Input: part model. Units: mm. Frame: model coordinates. A direction names the side the tool comes from. Round coordinates to 2 decimals unless told otherwise and drop trailing zeros. Write each loop counter-clockwise with the first axis right and the second up, starting at its lowest first coordinate (ties: lowest second). Pieces come first, ordered by that corner, then holes. Notation, with made-up numbers: (85, 24.25) -> (99, 24.25) arc R24 cw to (99, 52.25) -> close; hole circle Ø7 at (10.5, 23.5). An arc over 180 degrees is marked (long way). Write item = value, one per line.
Solid Edge part; units mm, degrees
sketch "Sketch1" plane through (0, 0, 0) normal (1, 0, 0) x (0, 1, 0)
  circle A0 centre (0, 0) radius 2.5
extrude "Protrusion1" add sketch "Sketch1" along normal mid plane 40
sketch "Sketch2" plane through (0, 0, 0) normal (0, -1, 0) x (1, 0, 0)
  line L0 (30, 0) -> (30, 20)
  line L1 (30, -10) -> (30, 0)
  line L2 (20, -10) -> (30, -10)
  line L3 (20, 20) -> (20, -10)
  line L4 (20, 20) -> (-20, 20)
  line L5 (-20, -10) -> (-20, 20)
  line L6 (-30, -10) -> (-20, -10)
  line L7 (-30, 0) -> (-30, -10)
  line L8 (-30, 20) -> (-30, 0)
  line L9 (-30, 30) -> (-30, 20)
  line L10 (30, 30) -> (-30, 30)
  line L11 (30, 20) -> (30, 30)
extrude "ExtrudedProtrusion_2" add sketch "Sketch2" along normal mid plane 10
sketch "Sketch3" plane through (0, -5, 10) normal (0, -1, 0) x (1, 0, 0)
  line L0 (-20, -20) -> (-20, -5)
  line L1 (-20, -5) -> (20, -5)
  line L2 (20, -5) -> (20, -20)
  line L3 (20, -20) -> (-20, -20)
extrude "ExtrudedCutout_1" cut sketch "Sketch3" against normal blind 16.4245
sketch "Sketch4" plane through (0, -5, 10) normal (0, -1, 0) x (1, 0, 0)
  line L0 (-30, -20) -> (-30, 20)
  line L1 (-30, 20) -> (30, 20)
  line L2 (30, 20) -> (30, -20)
  line L3 (30, -20) -> (20, -20)
  line L4 (20, -20) -> (20, 10)
  line L5 (20, 10) -> (-20, 10)
  line L6 (-20, 10) -> (-20, -20)
  line L7 (-20, -20) -> (-30, -20)
extrude "ExtrudedProtrusion_3" add sketch "Sketch4" along normal blind 30
sketch "Sketch5" plane through (30, -15, 10) normal (1, 0, 0) x (0, 1, 0)
  circle A0 centre (0, -5) radius 2.5
extrude "ExtrudedCutout_2" cut sketch "Sketch5" against normal blind 72.3648
fillet "Round_1" radius 10 4 edges at (-25, -35, -10) (25, -35, -10) (-25, 5, -10) (25, 5, -10)
sketch "Sketch6" plane through (0, -15, 30) normal (0, 0, 1) x (-1, 0, 0)
  line L0 (-30, -20) -> (-30, -10)
  line L1 (-30, -10) -> (30, -10)
  line L2 (30, -10) -> (30, -20)
  line L3 (30, -20) -> (-30, -20)
extrude "ExtrudedProtrusion_4" add sketch "Sketch6" along normal blind 210
sketch "Sketch7" plane through (0, -5, 135) normal (0, -1, 0) x (0, 0, 1)
  line L0 (105, -30) -> (95, -30)
  line L1 (95, -30) -> (95, 30)
  line L2 (95, 30) -> (105, 30)
  line L3 (105, 30) -> (105, -30)
extrude "Protrusion2" add sketch "Sketch7" along normal up to vertex (30 mm away)
sketch "Sketch8" plane through (30, -15, 115) normal (1, 0, 0) x (0, 0, 1)
  line L0 (-85, 20) -> (-95, 20)
  line L1 (-95, 20) -> (-95, -20)
  line L2 (-95, -20) -> (125, -20)
  line L3 (125, -20) -> (125, 20)
  line L4 (125, 20) -> (115, 20)
  line L5 (115, 20) -> (115, -10)
  line L6 (115, -10) -> (-85, -10)
  line L7 (-85, -10) -> (-85, 20)
extrude "ExtrudedProtrusion_6" add sketch "Sketch8" along normal blind 100
sketch "Sketch9" plane through (-30, -15, 115) normal (-1, 0, 0) x (0, 0, -1)
  line L0 (-125, 20) -> (-125, -20)
  line L1 (95, -20) -> (-125, -20)
  line L2 (95, 20) -> (95, -20)
  line L3 (85, 20) -> (95, 20)
  line L4 (85, -10) -> (85, 20)
  line L5 (-115, -10) -> (85, -10)
  line L6 (-115, 20) -> (-115, -10)
  line L7 (-125, 20) -> (-115, 20)
extrude "ExtrudedProtrusion_7" add sketch "Sketch9" along normal blind 100
sketch "Sketch10" plane through (0, -5, 130) normal (0, -1, 0) x (1, 0, 0)
  line L0 (-130, 100) -> (-120, 100)
  line L1 (-120, 100) -> (-120, -100)
  line L2 (-120, -100) -> (-130, -100)
  line L3 (-130, -100) -> (-130, 100)
  line L4 (130, 100) -> (120, 100)
  line L5 (120, 100) -> (120, -100)
  line L6 (120, -100) -> (130, -100)
  line L7 (130, -100) -> (130, 100)
extrude "ExtrudedProtrusion_8" add sketch "Sketch10" along normal blind 30
fillet "Round_2" radius 10 4 edges at (-30, -15, 20) (30, -15, 20) (-20, -15, 20) (20, -15, 20)
sketch "Sketch11" plane through (0, 5, 120) normal (0, 1, 0) x (0, 0, -1)
  line L0 (-40, 130) -> (-10, 130)
  line L1 (-10, 130) -> (20, 130)
  line L2 (20, 130) -> (20, 100)
  line L3 (20, 100) -> (-40, 100)
  line L4 (-40, 100) -> (-40, 130)
  line L5 (-40, -130) -> (-40, -100)
  line L6 (-40, -100) -> (20, -100)
  line L7 (20, -100) -> (20, -130)
  line L8 (20, -130) -> (-40, -130)
extrude "ExtrudedCutout_3" cut sketch "Sketch11" against normal blind 1
1) Line query: L1, parallel to Z at x = -22, y = -15; L2, parallel to X at y = -28.5, z = 108; L3, parallel to Y at x = -50, z = 204. Output: solid intervals per line, ascending. Write a range as from..to.
Solutions:
L1 = -10..2.5, 7.5..30, 230..240
L2 = -130..-120, 120..130
L3 = -5..5
2) Access query for faces 1 (the face through (84, -15, 20)), 2 (the face through (-120, -20, 131)), 3 (the face through (17.15, -15.28, 16.99)). Directions: +Z, -Z, +X, -X, +Y, -Y. A direction counts if a zero-diameter tool reaches every point of the face in a straight line with its end or side. Return the directions, or none.
Solutions:
face_1 = -Z, +X, +Y, -Y
face_2 = -Y
face_3 = -Z, +Y, -Y
3) Draft query along X for faces 4 (the face through (-30, -15, 0)), 5 (the face through (130, -15, 128)), 6 (the face through (25.07, 1.99, -7.15)), 7 (the face through (-16.99, -15.28, 17.15)). Return one class per face: +X half, -X half, draft (parallel to the pull), parting line (faces both ways), or undercut.
Solutions:
face_4 = -X half
face_5 = +X half
face_6 = draft
face_7 = undercut
4) First-contact query: P1, Ø8, axis at x = -76, y = -25, coming from the -Z side; P2, Ø15, axis at x = -109.5, z = 127, coming from the +Y side; P3, Ø4.5, axis at y = -15, z = 5, coming from the +X side; P4, Ø22, axis at y = -23.5, z = 3.5, coming from the +X side. Flat tips, straight axial feed; report the tip coordinate or a pass-through.
Solutions:
P1 = 20
P2 = 4
P3 = through
P4 = 31.07
5) Cut plane D-D (z = 41.5). Return the cut outline in (x, y).
Solutions:
outline = (-130, -35) -> (-120, -35) -> (-120, -5) -> (120, -5) -> (120, -35) -> (130, -35) -> (130, 5) -> (-130, 5) -> close
6) Cut plane C-C (y = 1). Return the cut outline in (x, z).
Solutions:
outline = (-130, 20) -> (-40, 20) arc R10 cw to (-30, 10) -> (-30, -8) -> (-20, -8) -> (-20, 10) arc R10 cw to (-10, 20) -> (10, 20) arc R10 cw to (20, 10) -> (20, -8) -> (30, -8) -> (30, 10) arc R10 cw to (40, 20) -> (130, 20) -> (130, 240) -> (-130, 240) -> close
7) Cut plane B-B (x = -109.5). Return the cut outline in (y, z), and give its area (3 significant figures).
Solutions:
outline = (-35, 20) -> (5, 20) -> (5, 100) -> (4, 100) -> (4, 160) -> (5, 160) -> (5, 240) -> (-35, 240) -> (-35, 230) -> (-5, 230) -> (-5, 30) -> (-35, 30) -> close
area = 2,740 mm^2
8) Cut plane A-A (y = -22). Return the cut outline in (x, z).
Solutions:
outline = (-130, 20) -> (-40, 20) arc R10 cw to (-30, 10) -> (-30, -10) -> (-20, -10) -> (-20, 10) arc R10 cw to (-10, 20) -> (10, 20) arc R10 cw to (20, 10) -> (20, -10) -> (30, -10) -> (30, 10) arc R10 cw to (40, 20) -> (130, 20) -> (130, 240) -> (-130, 240) -> close; hole (-120, 30) -> (120, 30) -> (120, 230) -> (-120, 230) -> close
